```python
from build123d import *

# Parameters (mm, degrees)
HOLE_WIZARD_M21_D           = 2.4
HOLE_WIZARD_M21_CSINK_D     = 4.4
HOLE_WIZARD_M21_CSINK_ANGLE = 90
PATTERN_CIRCULAR_1_COUNT    = 8


with BuildPart() as part:
    # Эскиз1 → Повернуть1 (revolve)
    with BuildSketch(Plane.XY):
        Polygon((0, 19), (0, 25), (1, 26), (3, 26), (3, 19), align=None)
    revolve(axis=Axis((0, 0, 0), (1, 0, 0)))

    # Зенковка для винта с потайной головкой M21 (through all)
    with Locations(Plane.ZY):
        with Locations((16.263455967, 16.263455967)):
            hole_wizard_m21 = CounterSinkHole(HOLE_WIZARD_M21_D / 2, HOLE_WIZARD_M21_CSINK_D / 2, counter_sink_angle=HOLE_WIZARD_M21_CSINK_ANGLE)

    # Круговой массив1: Зенковка для винта с потайной головкой M21 ×8 about axis
    pattern_circular_1_axis = Axis((0, 0, 0), (1, 0, 0))
    for i in range(1, PATTERN_CIRCULAR_1_COUNT):
        add(hole_wizard_m21.rotate(pattern_circular_1_axis, i * 360 / PATTERN_CIRCULAR_1_COUNT), mode=Mode.SUBTRACT)


solid = part.part
```
The listing builds one solid part. Answer for the finished solid, in the listing's coordinates (mm). Give positions to 0.01 mm unless a question says otherwise; leave off trailing zeros. Loops run counter-clockwise (first coordinate to the right, second up) from the corner with the lowest first, then second, coordinate; pieces in that order, holes last. Notation, with made-up numbers: (62.25, 4) - (96.25, 4) arc R25 ccw to (96.25, 20) - close; hole circle Ø8 at (85, 40.25). An arc over 180 degrees is marked (long way). Return JSON: item names as keys, results as strings. Group by question number.
1. Straight lines are drawn through the part: line 1 (Z direction, x = 2.65, y = 0); line 2 (Y direction, x = 2.95, z = -15.5); line 3 (Z direction, x = 2.35, y = 23). For each, find the intervals that lie inside material, in ascending order. Write a range as [from, to].
2. Given pin 1 Ø2 at (y, z) = (-16.26, 16.26) entering from +X; pin 2 Ø4 at (y, z) = (16.26, 16.26) entering from -X; pin 3 Ø3 at (y, z) = (23, 0) entering from -X, each flat-ended and moving along its own axis, determine where each tip first touches the part or whether it passes through.
3. Find section C-C (x = 1.65). State how many separate pieces and enclosed holes the cut face has, then the cut area to 3 significant figures.
4. Find section A-A (y = 0). Write down the section's boundary in (x, z).
5. Determine the mould class of faces 1 (the cylindrical face through (2.014, -15.533, -17.216)), 2 (the cylindrical face through (2.014, -20.633, -15.821)) for opening direction Y: pulls with the +Y half, pulls with the -Y half, needs draft (parallel to the pull), parting line crosses it, or undercut.
Verdict:
{
 "1": {"line 1": "z = [-26, -24.2], [-21.8, -19], [19, 21.8], [24.2, 26]", "line 2": "y = [-20.87, -17.19], [-15.34, -10.99], [10.99, 15.34], [17.19, 20.87]", "line 3": "z = [-12.12, -1.2], [1.2, 12.12]"},
 "2": {"pin 1": "passes through", "pin 2": "stops at x = 0.2", "pin 3": "stops at x = 0.7"},
 "3": {"separate pieces": "1", "enclosed holes": "9", "area": "953 mm^2"},
 "4": {"outline": "(0, -20.8) - (1, -21.8) - (3, -21.8) - (3, -19) - (0, -19) - close; (0, 19) - (3, 19) - (3, 21.8) - (1, 21.8) - (0, 20.8) - close; (0.1, -25.1) - (1, -26) - (3, -26) - (3, -24.2) - (1, -24.2) - close; (0.1, 25.1) - (1, 24.2) - (3, 24.2) - (3, 26) - (1, 26) - close"},
 "5": {"face 1": "undercut", "face 2": "parting line crosses it"}
}
